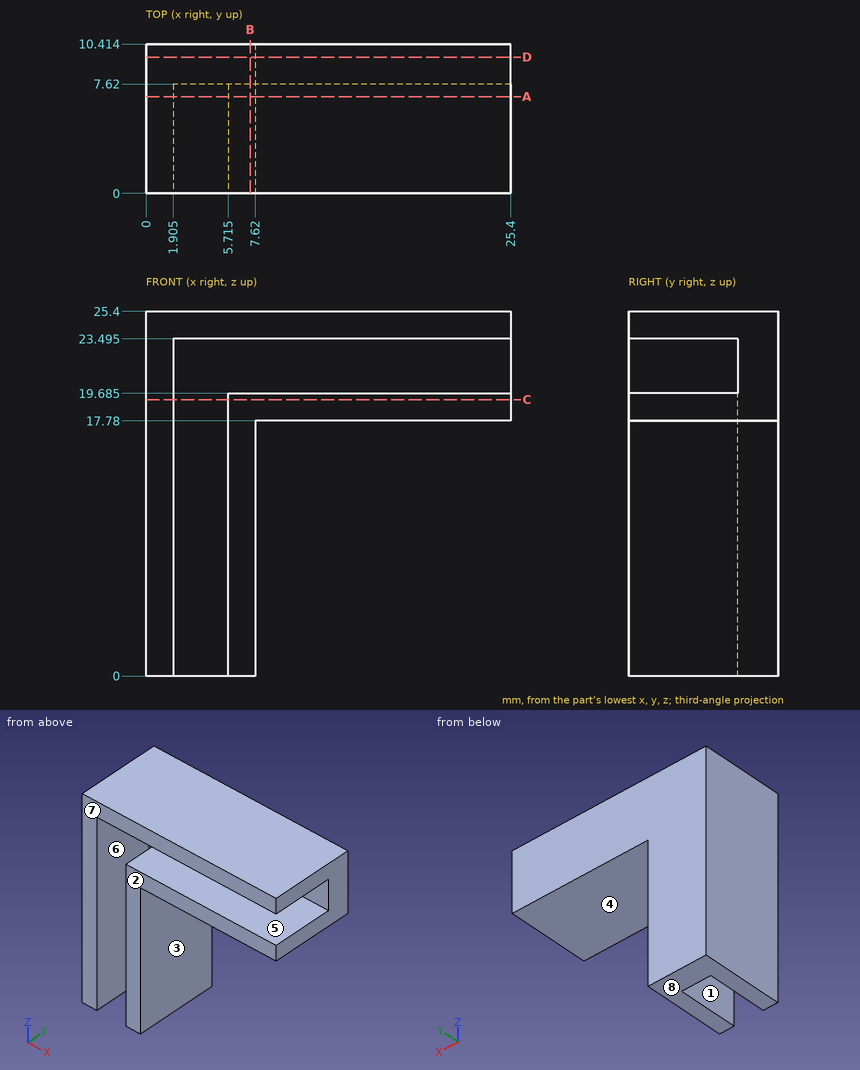
Answer from the drawing. Dimensions are ordinates in mm from the lowest x, y and z of the part. A direction names the side the tool comes from. Coordinates: 2 decimals unless noted, no trailing zeros. Order: outer loops, then holes, each group sorted by start corner. A loop starts at its lowest first (then second) coordinate and runs counter-clockwise, first axis right, second up. Notation, with made-up numbers: (-22, 80) - (-5, 80) arc R26 cw to (-5, 115) - close; hole circle Ø6 at (22, -14). An arc over 180 degrees is marked (long way). Answer as a JSON object with one key per item and string values. Group by question number.
Item 1: Section B-B (x = 7.25) is taken. Give the vertices of the cut face in (y, z) (3 decimals), plus the area to 3 significant figures.
Item 2: The mould has two halves that part along X. Classify the marked faces 1, 2 and 3: +X half, -X half, draft (parallel to the pull), parting line (faces both ways), or undercut.
Item 3: Flat-ended cylindrical pins translate along their axes: P1, Ø3, axis at y = 7.5, z = 7, coming from the +X side; P2, Ø1, axis at x = 22, z = 21, coming from the -Y side. Find the tip coordinate at first contact, or state that the pin passes through.
Item 4: Consider probe 1 along X at (y, z) = (1, 1) (3 decimals); probe 2 along Z at (x, y) = (6.5, 5.25) (3 decimals); probe 3 along Z at (x, y) = (17.75, 3.5) (3 decimals). Determine where each line is inside the solid, lowest interval first. Write a range as from..to.
Item 5: A tool of negligible diameter and unlimited length cuts with its end or side. For the marked faces 4, 5, 6, 7 and 8, from which of +Z, -Z, +X, -X, +Y, -Y can it reach the whole face along a straight path? Write none if from no direction.
Item 6: Section D-D (y = 9.5) is taken. Give the vertices of the cut face in (x, z).
Item 7: Section A-A (y = 6.75) is taken. Give the vertices of the cut face in (x, z) (3 decimals), plus the area to 3 significant figures.
Item 8: Section C-C (z = 19.25) is taken. Give the vertices of the cut face in (x, y) (3 decimals), plus the area to 3 significant figures.
Results are:
{
 "1": {"outline": "(0, 0) - (10.414, 0) - (10.414, 25.4) - (0, 25.4) - (0, 23.495) - (7.62, 23.495) - (7.62, 19.685) - (0, 19.685) - close", "area": "235 mm^2"},
 "2": {"face 1": "undercut", "face 2": "draft", "face 3": "+X half"},
 "3": {"P1": "stops at x = 7.62", "P2": "stops at y = 7.62"},
 "4": {"probe 1": "x = 0..1.905, 5.715..7.62", "probe 2": "z = 0..19.685, 23.495..25.4", "probe 3": "z = 17.78..19.685, 23.495..25.4"},
 "5": {"face 4": "-Z, +X, +Y, -Y", "face 5": "+X, -Y", "face 6": "-Z, -Y", "face 7": "+Z, -Z, +X, -X, -Y", "face 8": "-Z, +X, -X, +Y, -Y"},
 "6": {"outline": "(0, 0) - (7.62, 0) - (7.62, 17.78) - (25.4, 17.78) - (25.4, 25.4) - (0, 25.4) - close"},
 "7": {"outline": "(0, 0) - (1.905, 0) - (1.905, 23.495) - (25.4, 23.495) - (25.4, 25.4) - (0, 25.4) - close; (5.715, 0) - (7.62, 0) - (7.62, 17.78) - (25.4, 17.78) - (25.4, 19.685) - (5.715, 19.685) - close", "area": "165 mm^2"},
 "8": {"outline": "(0, 0) - (1.905, 0) - (1.905, 7.62) - (5.715, 7.62) - (5.715, 0) - (25.4, 0) - (25.4, 10.414) - (0, 10.414) - close", "area": "235 mm^2"}
}
